from build123d import *

# Parameters (mm, degrees)
BOSS_EXTRUDE1_DEPTH = 25.4
CUT_EXTRUDE1_DEPTH  = 12.7


with BuildPart() as part:
    # Sketch1 → Boss-Extrude1 (new, symmetric)
    with BuildSketch(Plane(origin=(0, 0, 0), x_dir=(0, 0, -1), z_dir=(1, 0, 0))):
        Polygon((7.332348419, 0), (3.666174209, 6.35), (-3.666174209, 6.35), (-7.332348419, 0), (-3.666174209, -6.35), (3.666174209, -6.35), align=None)
    extrude(amount=BOSS_EXTRUDE1_DEPTH, both=True)

    # Sketch2 → Cut-Extrude1 (cut)
    with BuildSketch(Plane.ZY.offset(25.4)):
        Polygon((3.464101579, 0), (1.73205079, 2.999999969), (-1.73205079, 2.999999969), (-3.464101579, 0), (-1.73205079, -2.999999969), (1.73205079, -2.999999969), align=None)
    extrude(amount=-CUT_EXTRUDE1_DEPTH, mode=Mode.SUBTRACT)


solid = part.part
Input: part model. Units: mm. Frame: model coordinates. A direction names the side the tool comes from. Coordinates: 2 decimals unless noted, no trailing zeros. Loops run counter-clockwise (first coordinate to the right, second up) from the corner with the lowest first, then second, coordinate; pieces in that order, holes last.
(1) First-contact query: pin 1 Ø2 at (x, z) = (6.5, -5.5) entering from -Y; pin 2 Ø1.5 at (x, z) = (15, 4.5) entering from -Y. Flat tips, straight axial feed; report the tip coordinate or a pass-through.
(2) Material intervals for probe 1 along Z at (x, y) = (-19.5, 1.75); probe 2 along X at (y, z) = (0, -2); probe 3 along Y at (x, z) = (-17, -2.5), sorted ascending.
(3) Section A-A on x = -16.5. Return the cut outline in (y, z), then the cut area to 3 significant figures.
(4) Section D-D on x = -1.5. Return the cut outline in (y, z), then the cut area to 3 significant figures.
(5) Section B-B on z = 1. Return the cut outline in (x, y).
(6) Section C-C on y = -2.5. Return the cut outline in (x, z), then the cut area to 3 significant figures.
(7) Set-up query: faces 1 (the face through (0.356, 3.131, -5.525)), 2 (the face through (-19.1, 1.5, -2.6)). Return all of +Z, -Z, +X, -X, +Y, -Y with unobstructed straight access to the full face (end or side cutting, diameter ignored); none if empty.
(8) Pull-direction query (Z, two-part tool) for faces 3 (the face through (-19.1, 1.5, 2.6)), 4 (the face through (25.4, 0, 0)), 5 (the face through (0.356, -3.131, 5.525)); classes: released by +Z, released by -Z, zero draft, split by the parting line, or undercut.
Data:
1. pin 1: stops at y = -4.91
1. pin 2: stops at y = -6.2
2. probe 1: z = -6.32 to -2.45, 2.45 to 6.32
2. probe 2: x = -12.7 to 25.4
2. probe 3: y = -6.35 to -1.67, 1.67 to 6.35
3. outline: (-6.35, -3.67) - (0, -7.33) - (6.35, -3.67) - (6.35, 3.67) - (0, 7.33) - (-6.35, 3.67) - close; hole (-3, -1.73) - (0, -3.46) - (3, -1.73) - (3, 1.73) - (0, 3.46) - (-3, 1.73) - close
3. area: 109 mm2
4. outline: (-6.35, -3.67) - (0, -7.33) - (6.35, -3.67) - (6.35, 3.67) - (0, 7.33) - (-6.35, 3.67) - close
4. area: 140 mm2
5. outline: (-25.4, -6.35) - (25.4, -6.35) - (25.4, 6.35) - (-25.4, 6.35) - (-25.4, 3) - (-12.7, 3) - (-12.7, -3) - (-25.4, -3) - close
6. outline: (-25.4, -5.89) - (25.4, -5.89) - (25.4, 5.89) - (-25.4, 5.89) - (-25.4, 2.02) - (-12.7, 2.02) - (-12.7, -2.02) - (-25.4, -2.02) - close
6. area: 547 mm2
7. face 1: -Z, +X, -X, +Y
7. face 2: -X
8. face 3: undercut
8. face 4: zero draft
8. face 5: released by +Z
